Verification items for this drawing (mm, ordinates from the low corner). A direction names the side the tool comes from. Round coordinates to 2 decimals unless told otherwise and drop trailing zeros. Order: outer loops, then holes, each group sorted by start corner. A loop starts at its lowest first (then second) coordinate and runs counter-clockwise, first axis right, second up. Notation, with made-up numbers: (-34, 7) - (-13, 7) arc R11 cw to (-13, 28) - close; hole circle Ø6 at (9.25, 76.25). An arc over 180 degrees is marked (long way). Return JSON: item names as keys, results as strings. Group by question number.
Q1. Material ranges on line 1 along Z through (x, y) = (9.9, 0.85); line 2 along Y through (x, z) = (8.5, 13.5); line 3 along X through (y, z) = (8, 11) (1 decimal), recorded low to high.
Q2. Sectioned sample at C-C, the plane x = 31.5. Record the cut outline in (y, z), then the cut area to 3 significant figures.
Q3. Tool access check on the marked faces 1 and 2. Record the directions out of +Z, -Z, +X, -X, +Y, -Y that give a thin tool (end or side, any length) a straight path to the whole face; none if there is none.
Q4. Gauge pin test, flat ends, axial feed: pin 1 Ø1.8 at (y, z) = (1, 22.5) entering from -X; pin 2 Ø0.8 at (y, z) = (0.5, 0.5) entering from -X; pin 3 Ø1.5 at (x, y) = (26, 7.5) entering from -Z; pin 4 Ø1.3 at (x, y) = (3.5, 0.5) entering from +Z. Record the tip position at first contact, or that the pin passes through.
Q5. Sectioned sample at A-A, the plane x = 9.9. Record the cut outline in (y, z).
Q6. Sectioned sample at B-B, the plane z = 11.9. Record the cut outline in (x, y).
Q7. Sectioned sample at D-D, the plane x = 14.5. Record the cut outline in (y, z).
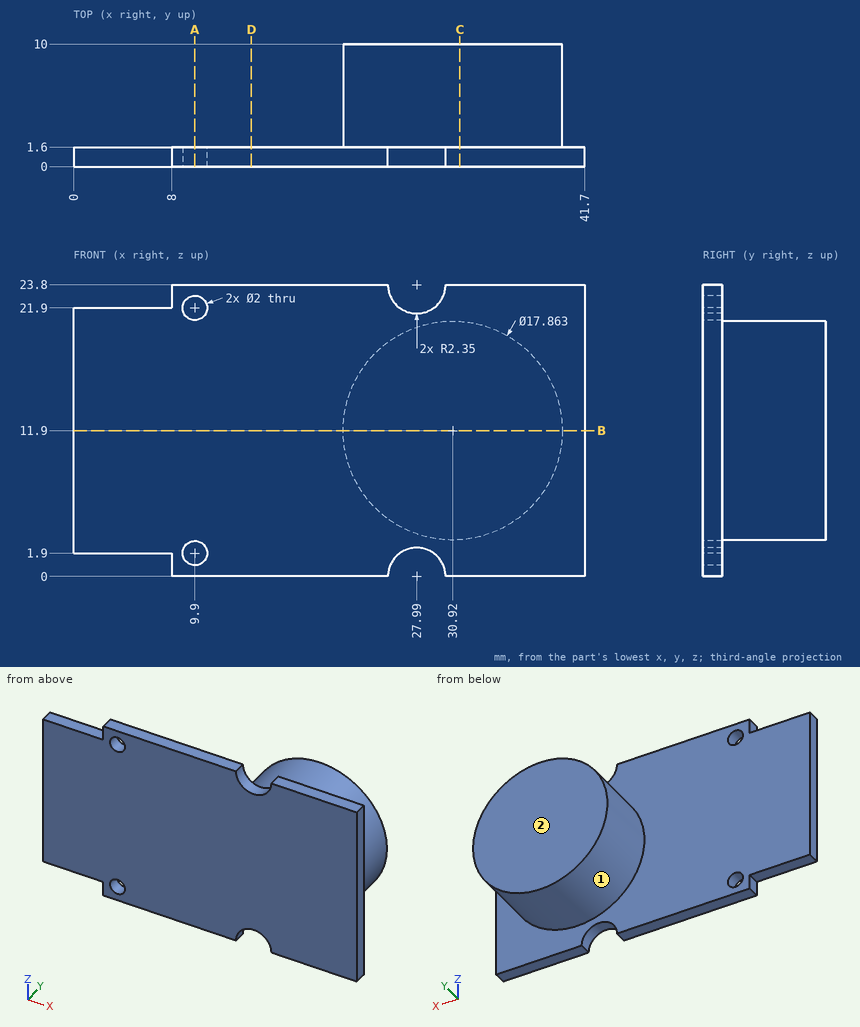
Reply:
{
 "1": {"line 1": "0 to 0.9, 2.9 to 20.9, 22.9 to 23.8", "line 2": "0 to 1.6", "line 3": "22 to 39.8"},
 "2": {"outline": "(0, 0) - (1.6, 0) - (1.6, 2.99) - (10, 2.99) - (10, 20.81) - (1.6, 20.81) - (1.6, 23.8) - (0, 23.8) - close", "area": "188 mm^2"},
 "3": {"face 1": "+Y", "face 2": "+Z, -Z, +X, -X, +Y"},
 "4": {"pin 1": "x = 0", "pin 2": "x = 8", "pin 3": "z = 4", "pin 4": "z = 21.9"},
 "5": {"outline": "(0, 0) - (1.6, 0) - (1.6, 0.9) - (0, 0.9) - close; (0, 2.9) - (1.6, 2.9) - (1.6, 20.9) - (0, 20.9) - close; (0, 22.9) - (1.6, 22.9) - (1.6, 23.8) - (0, 23.8) - close"},
 "6": {"outline": "(0, 0) - (41.7, 0) - (41.7, 1.6) - (39.85, 1.6) - (39.85, 10) - (21.99, 10) - (21.99, 1.6) - (0, 1.6) - close"},
 "7": {"outline": "(0, 0) - (1.6, 0) - (1.6, 23.8) - (0, 23.8) - close"}
}
